The listing builds one solid part. Answer for the finished solid, in the listing's coordinates (mm). A direction names the side the tool comes from. Give positions to 0.01 mm unless a question says otherwise; leave off trailing zeros. Order: outer loops, then holes, each group sorted by start corner. A loop starts at its lowest first (then second) coordinate and runs counter-clockwise, first axis right, second up. Notation, with made-up numbers: (66.5, 70.5) - (114.5, 70.5) arc R26 ccw to (114.5, 109.5) - close; hole circle Ø2 at (1.25, 67). An arc over 180 degrees is marked (long way). Answer as a JSON object with one key per item and string values. Group by question number.
Q1. Given pin 1 (4 mm diameter, centred on x = -3.5, y = -6.25, fed in from +Z); pin 2 (4 mm diameter, centred on y = -2, z = 15.5, fed in from -X); pin 3 (1 mm diameter, centred on x = 2.5, z = 15.5, fed in from -Y); pin 4 (10.5 mm diameter, centred on x = 14, y = -6.5, fed in from +Z), each flat-ended and moving along its own axis, determine where each tip first touches the part or whether it passes through.
Q2. A cutting plane is placed at D-D, the plane y = -9.75. Give the vertices of the cut face in (x, z).
Q3. The mould has two halves that part along X. Classify faces 1 (the face through (9.608, -16.722, 12.375)), 2 (the face through (23.25, -8, 14)), 3 (the face through (10.3, -18.75, 13.6)): released by +X, released by -X, zero draft, split by the parting line, or undercut.
Q4. For faces 4 (the face through (-1.56, -16.72, 16.19)), 5 (the face through (11.1, -15, 17)), 6 (the face through (-2, -11, 13)), 7 (the face through (-1, -7.75, 13)), 8 (the face through (11, 0, 14)), determine the directions among +Z, -Z, +X, -X, +Y, -Y from which every point of the face is accessible in a straight line to the end or side of a thin tool.
Q5. A cutting plane is placed at B-B, the plane y = -6.25. Give the vertices of the cut face in (x, z), and give its area (3 significant figures).
Q6. A cutting plane is placed at C-C, the plane z = 10.5. Give the vertices of the cut face in (x, y), and give its area (3 significant figures).
Q7. Consider line 1 (X direction, y = -3.25, z = 11.25); line 2 (Y direction, x = 17, z = 14.25); line 3 (Y direction, x = 1, z = 14.5). Determine where each line is inside the solid, lowest interval first.
Q8. A cutting plane is placed at A-A, the plane x = -3.5. Give the vertices of the cut face in (y, z).
from build123d import *

# Parameters (mm, degrees)
SKETCH1_W           = 27.25
SKETCH1_H           = 16.75
SKETCH1_W_2         = 23.25
SKETCH1_H_2         = 12.75
BOSS_EXTRUDE1_DEPTH = 18
SKETCH3_W           = 23.25
SKETCH3_H           = 12.75
BOSS_EXTRUDE2_DEPTH = 2
SKETCH7_W           = 2
SKETCH7_H           = 5
CUT_EXTRUDE1_DEPTH  = 2
SKETCH10_W          = 23.25
SKETCH10_H          = 12.75
SKETCH10_W_2        = 7
SKETCH10_H_2        = 16.75
BOSS_EXTRUDE3_DEPTH = 2
SKETCH11_R          = 1.5
CUT_EXTRUDE3_DEPTH  = 2
SKETCH12_R          = 1.5
CUT_EXTRUDE4_DEPTH  = 2
FILLET11_R          = 1
SKETCH13_W          = 3
SKETCH13_H          = 16.75
CUT_EXTRUDE5_DEPTH  = 10
CUT_EXTRUDE6_REACH  = 41.193
SKETCH14_W          = 27.25
SKETCH14_H          = 8
SKETCH16_W          = 23.25
SKETCH16_H          = 2
BOSS_EXTRUDE5_DEPTH = 7.6
SKETCH19_W          = 2
SKETCH19_H          = 3
CUT_EXTRUDE8_DEPTH  = 10
BOSS_EXTRUDE6_DEPTH = 4
SKETCH21_R          = 1.25
CUT_EXTRUDE9_DEPTH  = 2
BOSS_EXTRUDE7_DEPTH = 1
CUT_EXTRUDE11_START = -12
CUT_EXTRUDE11_DEPTH = 12


with BuildPart() as part:
    # Sketch1 → Boss-Extrude1 (new body)
    with BuildSketch(Plane.XY):
        with Locations((11.625, -6.375)):
            Rectangle(SKETCH1_W, SKETCH1_H)
        with Locations((11.625, -6.375)):
            Rectangle(SKETCH1_W_2, SKETCH1_H_2, mode=Mode.SUBTRACT)
    extrude(amount=BOSS_EXTRUDE1_DEPTH)

    # Sketch3 → Boss-Extrude2 (add)
    with BuildSketch(Plane(origin=(0, 0, 0), x_dir=(-1, 0, 0), z_dir=(0, 0, -1))):
        with Locations((-11.625, -6.375)):
            Rectangle(SKETCH3_W, SKETCH3_H)
    extrude(amount=-BOSS_EXTRUDE2_DEPTH)

    # Sketch7 → Cut-Extrude1 (cut)
    with BuildSketch(Plane.ZY.offset(2)):
        with Locations((3, -6.5)):
            Rectangle(SKETCH7_W, SKETCH7_H)
    extrude(amount=-CUT_EXTRUDE1_DEPTH, mode=Mode.SUBTRACT)

    # Sketch10 → Boss-Extrude3 (add)
    # profile 1 of 3: a face of its own
    with BuildSketch(Plane.XY.offset(18)):
        Polygon((-2, -0.03961342), (-2, 2), (-9, 2), (-9, -14.75), (-2, -14.75), (-2, -13.03961342), align=None)
    # profile 2 of 3: a face of its own
    with BuildSketch(Plane.XY.offset(18)):
        Polygon((25.25, 2), (-2, 2), (-2, -0.03961342), (-2, -13.03961342), (-2, -14.75), (25.25, -14.75), align=None)
        with Locations((11.625, -6.375)):
            Rectangle(SKETCH10_W, SKETCH10_H, mode=Mode.SUBTRACT)
    # profile 3 of 3: a face of its own
    with BuildSketch(Plane.XY.offset(18)):
        with Locations((28.75, -6.375)):
            Rectangle(SKETCH10_W_2, SKETCH10_H_2)
    extrude(amount=BOSS_EXTRUDE3_DEPTH)

    # Sketch11 → Cut-Extrude3 (cut)
    with BuildSketch(Plane(origin=(0, 0, 18), x_dir=(-1, 0, 0), z_dir=(0, 0, -1))):
        with Locations((3.5, -6.25)):
            Circle(SKETCH11_R)
    extrude(amount=-CUT_EXTRUDE3_DEPTH, mode=Mode.SUBTRACT)

    # Sketch12 → Cut-Extrude4 (cut)
    with BuildSketch(Plane(origin=(0, 0, 18), x_dir=(-1, 0, 0), z_dir=(0, 0, -1))):
        with Locations((-26.95, -6.25)):
            Circle(SKETCH12_R)
    extrude(amount=-CUT_EXTRUDE4_DEPTH, mode=Mode.SUBTRACT)

    # Fillet11
    fillet11_edges = [part.edges().sort_by_distance(p)[0] for p in [
        (0, -9, 3),
        (0, -4, 3),
        (0, -6.5, 4),
        (-2, -6.5, 4),
        (-2, -4, 3),
        (-2, -9, 3),
    ]]
    fillet(fillet11_edges, radius=FILLET11_R - 0.0001)  # a hair under: the kernel refuses the full size

    # Sketch13 → Cut-Extrude5 (cut)
    with BuildSketch(Plane(origin=(0, 0, 18), x_dir=(-1, 0, 0), z_dir=(0, 0, -1))):
        with Locations((-30.75, -6.375)):
            Rectangle(SKETCH13_W, SKETCH13_H)
        with Locations((7.5, -6.375)):
            Rectangle(SKETCH13_W, SKETCH13_H)
    extrude(amount=-CUT_EXTRUDE5_DEPTH, mode=Mode.SUBTRACT)

    # Cut-Extrude6: up to this face of the body (flat: up to its plane)
    cut_extrude6_end = Plane(part.part.faces().sort_by_distance((11.625, -14.75, 10.256684492))[0])
    # Sketch14 → Cut-Extrude6 (cut, up to the picked face)
    with BuildSketch(Plane(origin=(0, 2, 0), x_dir=(1, 0, 0), z_dir=(0, 1, 0)), mode=Mode.PRIVATE) as cut_extrude6_sk1:
        with Locations((11.625, -4)):
            Rectangle(SKETCH14_W, SKETCH14_H)
    cut_extrude6_tool1 = split(extrude(cut_extrude6_sk1.sketch, amount=-CUT_EXTRUDE6_REACH, mode=Mode.PRIVATE), bisect_by=cut_extrude6_end, keep=Keep.BOTH, mode=Mode.PRIVATE)
    add(cut_extrude6_tool1.solids().sort_by(Axis((11.625, 2, 4), (0, -1, 0)))[0], mode=Mode.SUBTRACT)

    # Sketch16 → Boss-Extrude5 (add)
    with BuildSketch(Plane.XY.offset(20)):
        with Locations((11.625, -13.75)):
            Rectangle(SKETCH16_W, SKETCH16_H)
    extrude(amount=BOSS_EXTRUDE5_DEPTH)

    # Sketch19 → Cut-Extrude8 (cut)
    with BuildSketch(Plane(origin=(0, 0, 8), x_dir=(-1, 0, 0), z_dir=(0, 0, -1))):
        with Locations((1, -6.25)):
            Rectangle(SKETCH19_W, SKETCH19_H)
        with Locations((-24.25, -6.25)):
            Rectangle(SKETCH19_W, SKETCH19_H)
    extrude(amount=-CUT_EXTRUDE8_DEPTH, mode=Mode.SUBTRACT)

    # Sketch20 → Boss-Extrude6 (add)
    with BuildSketch(Plane.XZ.offset(14.75)):
        with BuildLine():
            ThreePointArc((1.734487906, 14.866457564), (-0.15, 17.000000025), (1.734487955, 19.133542442))
            Line((1.734487955, 19.133542442), (4.661486136, 19.497797339))
            ThreePointArc((4.661486136, 19.497797339), (3.240091566, 20.432881138), (1.549246975, 20.622060423))
            ThreePointArc((1.549246975, 20.622060423), (0.742054746, 20.4263791), (0, 20.053276928))
            Line((0, 20.053276928), (0, 20))
            Line((0, 20), (-0.079062289, 20))
            ThreePointArc((-0.079062289, 20), (-1.544419903, 16.128456799), (1.549246968, 13.377939578))
            ThreePointArc((1.549246968, 13.377939578), (3.240091563, 13.567118861), (4.661486136, 14.502202661))
            Line((4.661486136, 14.502202661), (1.734487906, 14.866457564))
        make_face()
        with BuildLine():
            ThreePointArc((1.549246975, 20.622060423), (3.240091566, 20.432881138), (4.661486136, 19.497797339))
            Line((4.661486136, 19.497797339), (14.257253364, 20.691957699))
            ThreePointArc((14.257253364, 20.691957699), (15.89224684, 22.015782374), (17.896084422, 22.656368345))
            Line((17.896084422, 22.656368345), (1.549246975, 20.622060423))
        make_face()
        with BuildLine():
            ThreePointArc((17.896084422, 22.656368345), (15.89224684, 22.015782374), (14.257253364, 20.691957699))
            Line((14.257253364, 20.691957699), (18.081325153, 21.167850334))
            ThreePointArc((18.081325153, 21.167850334), (21.380428532, 20.14789091), (22.8, 17))
            ThreePointArc((22.8, 17), (21.380428595, 13.852109147), (18.081325321, 12.832149645))
            Line((18.081325321, 12.832149645), (14.257253364, 13.308042301))
            ThreePointArc((14.257253364, 13.308042301), (15.89224684, 11.984217626), (17.896084422, 11.343631655))
            ThreePointArc((17.896084422, 11.343631655), (22.37343883, 12.727862432), (24.3, 17))
            ThreePointArc((24.3, 17), (24.082512903, 18.559503854), (23.446648326, 20))
            Line((23.446648326, 20), (23.25, 20))
            Line((23.25, 20), (23.25, 20.296589146))
            ThreePointArc((23.25, 20.296589146), (20.898920406, 22.215837897), (17.896084422, 22.656368345))
        make_face()
        with BuildLine():
            Line((14.257253364, 13.308042301), (4.661486136, 14.502202661))
            ThreePointArc((4.661486136, 14.502202661), (3.240091563, 13.567118861), (1.549246968, 13.377939578))
            Line((1.549246968, 13.377939578), (17.896084422, 11.343631655))
            ThreePointArc((17.896084422, 11.343631655), (15.89224684, 11.984217626), (14.257253364, 13.308042301))
        make_face()
    extrude(amount=BOSS_EXTRUDE6_DEPTH)

    # Sketch21 → Cut-Extrude9 (cut)
    with BuildSketch(Plane.XZ.offset(14.75)):
        with Locations((18.6, 17)):
            Circle(SKETCH21_R)
    extrude(amount=-CUT_EXTRUDE9_DEPTH, mode=Mode.SUBTRACT)

    # Sketch23 → Boss-Extrude7 (add)
    with BuildSketch(Plane.XZ.offset(14.75)):
        Polygon((11.1, 21.100651295), (0.406174607, 19.998863224), (-0.954500861, 17.320033397), (0.387681288, 14.425953139), (11.1, 12.86779769), align=None)
    extrude(amount=BOSS_EXTRUDE7_DEPTH)

    # Sketch24 → Cut-Extrude11 (cut)
    with BuildSketch(Plane.XZ.offset(14.75).offset(CUT_EXTRUDE11_START)):
        with BuildLine():
            ThreePointArc((0, 20.053276928), (0.742054739, 20.426379098), (1.549246961, 20.622060422))
            Line((1.549246961, 20.622060422), (17.896084422, 22.656368345))
            ThreePointArc((17.896084422, 22.656368345), (20.898920406, 22.215837897), (23.25, 20.296589146))
            Line((23.25, 20.296589146), (23.25, 27.6))
            Line((23.25, 27.6), (0, 27.6))
            Line((0, 27.6), (0, 20.053276928))
        make_face()
    extrude(amount=CUT_EXTRUDE11_DEPTH, mode=Mode.SUBTRACT)


solid = part.part
Reply:
{
 "1": {"pin 1": "stops at z = 20", "pin 2": "stops at x = -2", "pin 3": "stops at y = -15.75", "pin 4": "passes through"},
 "2": {"outline": "(-6, 18) - (-2, 18) - (-2, 8) - (0, 8) - (0, 20) - (-6, 20) - close; (23.25, 8) - (25.25, 8) - (25.25, 18) - (29.25, 18) - (29.25, 20) - (23.25, 20) - close"},
 "3": {"face 1": "released by -X", "face 2": "undercut", "face 3": "zero draft"},
 "4": {"face 4": "-X, -Y", "face 5": "-Y", "face 6": "-Z, -X, +Y, -Y", "face 7": "-Z, +X, -X", "face 8": "+Z, -Z"},
 "5": {"outline": "(-6, 18) - (-5, 18) - (-5, 20) - (-6, 20) - close; (-2, 18) - (0, 18) - (0, 20) - (-2, 20) - close; (23.25, 18) - (25.45, 18) - (25.45, 20) - (23.25, 20) - close; (28.45, 18) - (29.25, 18) - (29.25, 20) - (28.45, 20) - close", "area": "12.0 mm^2"},
 "6": {"outline": "(-2, -14.75) - (25.25, -14.75) - (25.25, -7.75) - (23.25, -7.75) - (23.25, -12.75) - (0, -12.75) - (0, -7.75) - (-2, -7.75) - close; (-2, -4.75) - (0, -4.75) - (0, 0) - (23.25, 0) - (23.25, -4.75) - (25.25, -4.75) - (25.25, 2) - (-2, 2) - close", "area": "148 mm^2"},
 "7": {"line 1": "x = -2 to 0, 23.25 to 25.25", "line 2": "y = -14.75 to -12.75, 0 to 2", "line 3": "y = -18.75 to -12.75, 0 to 2"},
 "8": {"outline": "(-14.75, 18) - (-7.75, 18) - (-7.75, 20) - (-14.75, 20) - close; (-4.75, 18) - (2, 18) - (2, 20) - (-4.75, 20) - close"}
}
